from build123d import *

# Parameters (mm, degrees)
AUFSATZ_LINEAR_AUSTRAGEN1_DEPTH  = 10
F_15_0_15_DURCHMESSER_BOHRUNG1_D = 15
SKIZZE8_W                        = 43
SKIZZE8_H                        = 43
SCHNITT_LINEAR_AUSTRAGEN2_DEPTH  = 10
M3_GEWINDEBOHRUNG1_D             = 2.5
M3_GEWINDEBOHRUNG1_DEPTH         = 8
M3_GEWINDEBOHRUNG1_CSINK_D       = 3.05
M3_GEWINDEBOHRUNG1_CSINK_ANGLE   = 90
M3_GEWINDEBOHRUNG1_TIP           = 0.751075774


with BuildPart() as part:
    # Skizze1 → Aufsatz-Linear austragen1 (new body)
    with BuildSketch(Plane(origin=(0, 0, 0), x_dir=(1, 0, 0), z_dir=(0, 1, 0))):
        with BuildLine():
            Line((-105, 90), (105, 90))
            ThreePointArc((105, 90), (112.071067812, 87.071067812), (115, 80))
            Line((115, 80), (115, 50))
            ThreePointArc((115, 50), (112.071067812, 42.928932188), (105, 40))
            Line((105, 40), (55, 40))
            ThreePointArc((55, 40), (44.393398282, 35.606601718), (40, 25))
            Line((40, 25), (40, -45))
            ThreePointArc((40, -45), (44.393398282, -55.606601718), (55, -60))
            Line((55, -60), (65, -60))
            ThreePointArc((65, -60), (72.071067812, -62.928932188), (75, -70))
            Line((75, -70), (75, -80))
            ThreePointArc((75, -80), (72.071067812, -87.071067812), (65, -90))
            Line((65, -90), (-65, -90))
            ThreePointArc((-65, -90), (-72.071067812, -87.071067812), (-75, -80))
            Line((-75, -80), (-75, -70))
            ThreePointArc((-75, -70), (-72.071067812, -62.928932188), (-65, -60))
            Line((-65, -60), (-55, -60))
            ThreePointArc((-55, -60), (-44.393398282, -55.606601718), (-40, -45))
            Line((-40, -45), (-40, 25))
            ThreePointArc((-40, 25), (-44.393398282, 35.606601718), (-55, 40))
            Line((-55, 40), (-105, 40))
            ThreePointArc((-105, 40), (-112.071067812, 42.928932188), (-115, 50))
            Line((-115, 50), (-115, 80))
            ThreePointArc((-115, 80), (-112.071067812, 87.071067812), (-105, 90))
        make_face()
    extrude(amount=AUFSATZ_LINEAR_AUSTRAGEN1_DEPTH)

    # Ø15.0 (15) Durchmesser Bohrung1 (through all)
    with Locations(Plane(origin=(0, 10, 0), x_dir=(1, 0, 0), z_dir=(0, 1, 0))):
        with Locations((-85, 65), (85, 65)):
            Hole(F_15_0_15_DURCHMESSER_BOHRUNG1_D / 2)

    # Skizze8 → Schnitt-Linear austragen2 (cut)
    with BuildSketch(Plane(origin=(0, 10, 0), x_dir=(1, 0, 0), z_dir=(0, 1, 0))):
        with Locations((0, 37)):
            Rectangle(SKIZZE8_W, SKIZZE8_H)
    extrude(amount=-SCHNITT_LINEAR_AUSTRAGEN2_DEPTH, mode=Mode.SUBTRACT)

    # M3 Gewindebohrung1
    with Locations(Plane(origin=(0, 10, 0), x_dir=(1, 0, 0), z_dir=(0, 1, 0))):
        with Locations((-29.5, 66.5), (-29.5, 7.5), (29.5, 7.5), (29.5, 66.5)):
            CounterSinkHole(M3_GEWINDEBOHRUNG1_D / 2, M3_GEWINDEBOHRUNG1_CSINK_D / 2, depth=M3_GEWINDEBOHRUNG1_DEPTH, counter_sink_angle=M3_GEWINDEBOHRUNG1_CSINK_ANGLE)
            with Locations((0, 0, -(M3_GEWINDEBOHRUNG1_DEPTH + M3_GEWINDEBOHRUNG1_TIP / 2))):  # 118° drill point
                Cone(0, M3_GEWINDEBOHRUNG1_D / 2, M3_GEWINDEBOHRUNG1_TIP, mode=Mode.SUBTRACT)


solid = part.part
Geometry check sheet. Reference: the model listing, model coordinates, mm. A direction names the side the tool comes from. Round coordinates to 2 decimals unless told otherwise and drop trailing zeros. Order: outer loops, then holes, each group sorted by start corner. A loop starts at its lowest first (then second) coordinate and runs counter-clockwise, first axis right, second up. Notation, with made-up numbers: M 41.25,41.25 L 71.25,41.25 A20 ccw 71.25,70.25 Z; hole C 83,-13.5 d2. An arc over 180 degrees is marked long. Answer in a Markdown table with one row per item.
(1) Sectioned sample at C-C, the plane z = -42.5. Record the cut outline in (x, y).
Responses:
| item | result |
|---|---|
| outline | M -111.61,0 L -21.5,0 L -21.5,10 L -111.61,10 Z; M 21.5,0 L 111.61,0 L 111.61,10 L 21.5,10 Z |
(2) Draft check along X on faces 6 (the face through (71.99, 4.93, 62.85)), 7 (the face through (-77.507, 4.93, -65.33)), 8 (the face through (-111.99, 4.93, -42.85)). Enter one of: released by +X, released by -X, zero draft, split by the parting line, or undercut.
Responses:
| item | result |
|---|---|
| face 6 | released by +X |
| face 7 | undercut |
| face 8 | released by -X |
(3) Go/stop test with flat-tipped pins: P1, Ø1.5, axis at y = 3.5, z = -2, coming from the +X side; P2, Ø5, axis at y = 3.5, z = -33, coming from the +X side; P3, Ø5, axis at y = 1.5, z = -3, coming from the -X side. Record where each tip stops, or that it passes through.
Responses:
| item | result |
|---|---|
| P1 | stops at x = 40 |
| P2 | stops at x = 44.29 |
| P3 | stops at x = -40 |
(4) Scan lines: probe 1 along X at (y, z) = (5.5, -7.5); probe 2 along X at (y, z) = (8, -65); probe 3 along Z at (x, y) = (29.5, 7.75). Record each from-to range of solid material in increasing order. Write a range as from..to.
Responses:
| item | result |
|---|---|
| probe 1 | x = -40..-30.75, -28.25..28.25, 30.75..40 |
| probe 2 | x = -115..-92.5, -77.5..77.5, 92.5..115 |
| probe 3 | z = -90..-67.75, -65.25..-8.75, -6.25..90 |
(5) Sectioned sample at D-D, the plane z = 25. Record the cut outline in (x, y), and give its area (3 significant figures).
Responses:
| item | result |
|---|---|
| outline | M -40,0 L 40,0 L 40,10 L -40,10 Z |
| area | 800 mm² |
(6) Tool access check on faces 1 (the face through (75, 5, 75)), 2 (the face through (-21.5, 5, -37)), 3 (the face through (60, 5, 60)), 4 (the face through (-44.28, 4.93, -35.49)), 5 (the face through (2, 10, -1)). Record the directions out of +Z, -Z, +X, -X, +Y, -Y that give a thin tool (end or side, any length) a straight path to the whole face; none if there is none.
Responses:
| item | result |
|---|---|
| face 1 | +Z, +X, +Y, -Y |
| face 2 | +Y, -Y |
| face 3 | +X, +Y, -Y |
| face 4 | -X, +Y, -Y |
| face 5 | +Z, -Z, +X, -X, +Y |
(7) Sectioned sample at B-B, the plane y = 7.75. State how many separate pieces and enclosed holes the cut face has, and give its area (3 significant figures).
Responses:
| item | result |
|---|---|
| separate pieces | 1 |
| enclosed holes | 7 |
| area | 21,800 mm² |
(8) Sectioned sample at A-A, the plane x = 85. Record the cut outline in (y, z).
Responses:
| item | result |
|---|---|
| outline | M 0,-90 L 10,-90 L 10,-72.5 L 0,-72.5 Z; M 0,-57.5 L 10,-57.5 L 10,-40 L 0,-40 Z |
